Design review of the part built by this model. Coordinates are the model's own, in mm. A direction names the side the tool comes from. Coordinates: 2 decimals unless noted, no trailing zeros. Loops run counter-clockwise (first coordinate to the right, second up) from the corner with the lowest first, then second, coordinate; pieces in that order, holes last. Notation, with made-up numbers: M 16,26 L 47,26 A33 cw 47,59 Z; hole C 14.5,59 d2. An arc over 180 degrees is marked long. Answer as a JSON object with one key per item and string values. Group by question number.
1. To check wall thickness, follow probe 1 along Y at (x, z) = (9.5, 3.75) (3 decimals); probe 2 along Y at (x, z) = (23.91, 3.9) (3 decimals); probe 3 along X at (y, z) = (9, 5.25). State the ranges of each line that lie inside material, in increasing order.
2. Consider section A-A (x = 35.7). State the section outline as (y, z) points (3 decimals), then the cut area to 3 significant figures.
3. Draft analysis for pull direction Y (two halves, no side actions). For faces 4 (the flat face through (17, -1.947, 4)), 5 (the flat face through (-0.1, 24.5, 10)), state which applies: +Y half, -Y half, draft (parallel to the pull), parting line (faces both ways), or undercut.
4. Consider section B-B (x = -23.88). State the section outline as (y, z) points (3 decimals), then the cut area to 3 significant figures.
5. Insertion check: pin 1 (2.5 mm diameter, centred on y = -17, z = 3.5, fed in from -X); pin 2 (5 mm diameter, centred on y = -8.5, z = 7.5, fed in from -X); pin 3 (0.7 mm diameter, centred on y = 15, z = 3.5, fed in from +X); pin 4 (3 mm diameter, centred on x = 35.7, y = 14.725, fed in from -Z). Each pin has a flat end and moves straight along its axis. Give the tip position at first contact, or say it passes through.
6. Consider section D-D (z = 7.5). State the section outline as (x, y) points (3 decimals).
7. Consider section C-C (x = 12). State the section outline as (y, z) points (3 decimals).
8. Machinability: for faces 1 (the flat face through (26, 20, 5)), 2 (the flat face through (29.4, 0, 8)), 3 (the cylindrical face through (23.29, 17.293, 1.726)), which of the approach directions +Z, -Z, +X, -X, +Y, -Y give a long, thin tool a straight path to every point of the face, cutting with its end or side? Answer none if there is none.
from build123d import *

# Parameters (mm, degrees)
F0_W      = 56.2999993563
F0_H      = 48.5499993563
F0_R      = 4.025
F1_DEPTH  = 2.5
F0_R_2    = 2.86
F0_R_3    = 1.525
F2_DEPTH  = 5
F0_W_2    = 58.7999993563
F0_H_2    = 50.5499993563
F3_DEPTH  = 10
F0_W_3    = 61.3999993563
F0_H_3    = 53.6499993563
F4_DEPTH  = 6
F5_DEPTH  = 3.5
F6_W      = 53.6499993563
F6_H      = 2.5
F8_DEPTH  = 10
F7_W      = 53.6499993563
F7_H      = 2.5
F9_DEPTH  = 10
F10_R     = 2
F11_R     = 2
F12_DEPTH = 2.5
F13_W     = 46.75
F13_H     = 1
F13_H_2   = 1.5
F14_DEPTH = 3.4
F15_W     = 2
F15_H     = 28
F15_H_2   = 20.5807207916
F15_W_2   = 21.8790904619
F15_H_3   = 2
F15_H_4   = 20
F15_W_3   = 2.5
F15_H_5   = 12.8300296441
F16_DEPTH = 2.4
F17_R     = 1


with BuildPart() as f1:
    # F0 (on Top) → F1 (new body)
    with BuildSketch(Plane.XY):
        Rectangle(F0_W, F0_H)
        with Locations((-23.88, -20.035)):
            Circle(F0_R, mode=Mode.SUBTRACT)
        with Locations((23.91, 20.085)):
            Circle(F0_R, mode=Mode.SUBTRACT)
    extrude(amount=F1_DEPTH)

    # F0 (on Top) → F2 (join)
    with BuildSketch(Plane.XY):
        with Locations((-23.88, -20.035)):
            Circle(F0_R)
        with Locations((-23.88, -20.035)):
            Circle(F0_R_2, mode=Mode.SUBTRACT)
        with Locations((-23.88, -20.035)):
            Circle(F0_R_2)
        with Locations((-23.88, -20.035)):
            Circle(F0_R_3, mode=Mode.SUBTRACT)
        with Locations((23.91, 20.085)):
            Circle(F0_R)
        with Locations((23.91, 20.085)):
            Circle(F0_R_2, mode=Mode.SUBTRACT)
        with Locations((23.91, 20.085)):
            Circle(F0_R_2)
        with Locations((23.91, 20.085)):
            Circle(F0_R_3, mode=Mode.SUBTRACT)
    extrude(amount=F2_DEPTH)

    # F0 (on Top) → F3 (join)
    with BuildSketch(Plane.XY):
        Rectangle(F0_W_2, F0_H_2)
        Rectangle(F0_W, F0_H, mode=Mode.SUBTRACT)
    extrude(amount=F3_DEPTH)

    # F0 (on Top) → F4 (join)
    with BuildSketch(Plane.XY):
        Rectangle(F0_W_3, F0_H_3)
        Rectangle(F0_W_2, F0_H_2, mode=Mode.SUBTRACT)
    extrude(amount=F4_DEPTH)

    # F0 (on Top) → F5 (cut)
    with BuildSketch(Plane.XY):
        with Locations((-23.88, -20.035)):
            Circle(F0_R_2)
        with Locations((-23.88, -20.035)):
            Circle(F0_R_3, mode=Mode.SUBTRACT)
        with Locations((23.91, 20.085)):
            Circle(F0_R_2)
        with Locations((23.91, 20.085)):
            Circle(F0_R_3, mode=Mode.SUBTRACT)
    extrude(amount=F5_DEPTH, mode=Mode.SUBTRACT)

    # F6 (on face) → F8 (join)
    with BuildSketch(Plane(origin=(-30.6999996781, 0, 0), x_dir=(0, -1, 0), z_dir=(-1, 0, 0))):
        with Locations((0, 1.25)):
            Rectangle(F6_W, F6_H)
    extrude(amount=F8_DEPTH)

    # F7 (on face) → F9 (join)
    with BuildSketch(Plane.YZ.offset(30.6999996781)):
        with Locations((0, 1.25)):
            Rectangle(F7_W, F7_H)
    extrude(amount=F9_DEPTH)

    # F10 (on face) + F11 (on face) → F12 (cut)
    with BuildSketch(Plane.XY.offset(2.5)):
        with Locations((-35.6999996781, 14.8249996781)):
            Circle(F10_R)
        with Locations((-35.6999996781, -14.8249996781)):
            Circle(F10_R)
    with BuildSketch(Plane.XY.offset(2.5)):
        with Locations((35.6999996781, 14.7250003219)):
            Circle(F11_R)
        with Locations((35.6999996781, -14.8249996781)):
            Circle(F11_R)
    extrude(amount=-F12_DEPTH, mode=Mode.SUBTRACT)

    # F13 (on face) → F14 (cut)
    with BuildSketch(Plane.XY.offset(10)):
        with Locations((3.5249996781, -24.7749996781)):
            Rectangle(F13_W, F13_H)
        with Locations((3.5249996781, -26.0249996781)):
            Rectangle(F13_W, F13_H_2)
    extrude(amount=-F14_DEPTH, mode=Mode.SUBTRACT)

    # F15 (on face) → F16 (join)
    with BuildSketch(Plane.XY.offset(2.5)):
        with Locations((-16.6158268005, 10.2749996781)):
            Rectangle(F15_W, F15_H)
        with Locations((-11.205850333, 10.2749996781)):
            Rectangle(F15_W, F15_H)
        with Locations((-5.5801804885, 10.2749996781)):
            Rectangle(F15_W, F15_H)
        with Locations((15.2583353445, 13.9846392823)):
            Rectangle(F15_W, F15_H_2)
        with Locations((17.2104544472, -0.9468855462)):
            Rectangle(F15_W_2, F15_H_3)
        with Locations((14.4178884327, -14.2749996781)):
            Rectangle(F15_W, F15_H_4)
        with Locations((19.7637628987, -14.2749996781)):
            Rectangle(F15_W, F15_H_4)
        with Locations((24.7685218453, -14.2749996781)):
            Rectangle(F15_W, F15_H_4)
        with Locations((-1.164972987, -17.8599848561)):
            Rectangle(F15_W_3, F15_H_5)
    extrude(amount=F16_DEPTH)

    # F17
    f17_edges = [f1.edges().sort_by_distance(p)[0] for p in [
        (-40.7, 0, 2.5),
        (40.7, 0, 2.5),
        (-35.7, 26.825, 2.5),
        (-35.7, -26.825, 2.5),
        (35.7, -26.825, 2.5),
        (35.7, 26.825, 2.5),
    ]]
    fillet(f17_edges, radius=F17_R)


solid = f1.part
Findings below:
{
 "1": {"probe 1": "y = -26.825 to -24.275, -1.947 to 0.053, 24.275 to 26.825", "probe 2": "y = -26.825 to -4.275, -1.947 to 0.053, 16.06 to 18.56, 21.61 to 24.11, 24.275 to 26.825", "probe 3": "x = -30.7 to -28.15, 28.15 to 30.7"},
 "2": {"outline": "M -26.825,0 L -16.825,0 L -16.825,2.5 L -25.825,2.5 A1 ccw -26.825,1.5 Z; M -12.825,0 L 12.725,0 L 12.725,2.5 L -12.825,2.5 Z; M 16.725,0 L 26.825,0 L 26.825,1.5 A1 ccw 25.825,2.5 L 16.725,2.5 Z", "area": "114 mm^2"},
 "3": {"face 4": "undercut", "face 5": "draft"},
 "4": {"outline": "M -26.825,0 L -22.895,0 L -22.895,3.5 L -21.56,3.5 L -21.56,5 L -24.06,5 L -24.06,2.5 L -24.275,2.5 L -24.275,10 L -25.275,10 L -25.275,6 L -26.825,6 Z; M -18.51,3.5 L -17.175,3.5 L -17.175,0 L 26.825,0 L 26.825,6 L 25.275,6 L 25.275,10 L 24.275,10 L 24.275,2.5 L -16.01,2.5 L -16.01,5 L -18.51,5 Z", "area": "156 mm^2"},
 "5": {"pin 1": "stops at x = -40.36", "pin 2": "stops at x = -30.7", "pin 3": "stops at x = 30.7", "pin 4": "passes through"},
 "6": {"outline": "M -29.4,-25.275 L -19.85,-25.275 L -19.85,-24.275 L -28.15,-24.275 L -28.15,24.275 L 28.15,24.275 L 28.15,-24.275 L 26.9,-24.275 L 26.9,-25.275 L 29.4,-25.275 L 29.4,25.275 L -29.4,25.275 Z"},
 "7": {"outline": "M -26.825,0 L 26.825,0 L 26.825,6 L 25.275,6 L 25.275,10 L 24.275,10 L 24.275,2.5 L 0.053,2.5 L 0.053,4.9 L -1.947,4.9 L -1.947,2.5 L -24.275,2.5 L -24.275,6.6 L -25.275,6.6 L -25.275,6 L -26.825,6 Z"},
 "8": {"face 1": "+Z", "face 2": "+Z, +X, +Y, -Y", "face 3": "-Z"}
}
